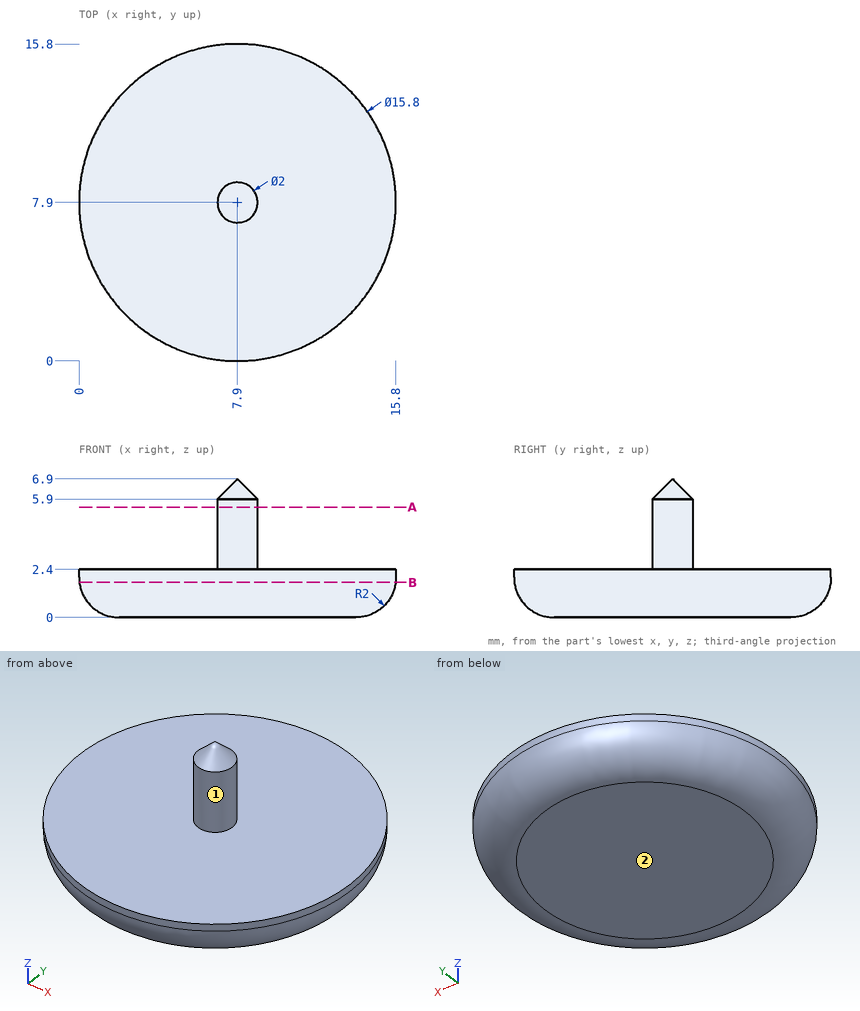
Design review of the part shown in the three views and the two pictorial views. Dimensions are in mm from the part's minimum x, y and z. A direction names the side the tool comes from. Round coordinates to 2 decimals unless told otherwise and drop trailing zeros. Loops run counter-clockwise (first coordinate to the right, second up) from the corner with the lowest first, then second, coordinate; pieces in that order, holes last. Notation, with made-up numbers: (37.5, -34.5) -> (71.5, -34.5) arc R30 cw to (71.5, -9.5) -> close; hole circle Ø10 at (26, 27.25). An arc over 180 degrees is marked (long way). Return JSON: item names as keys, results as strings.
(1) For pin 1 (3 mm diameter, centred on x = 13.5, y = 8.5, fed in from +Z); pin 2 (6 mm diameter, centred on x = 5, y = 2, fed in from -Z), all flat-tipped, find the tip position at first contact; note any pin that passes through.
Solved:
{"pin 1": "z = 2.4", "pin 2": "z = 0"}
(2) Add section B-B on z = 1.75. Write out the cut boundary in (x, y).
Solved:
{"outline": "circle Ø15.77 at (7.9, 7.9)"}
(3) For line 1 (Z direction, x = 9.25, y = 9.25); line 2 (X direction, y = 9.5, z = 1.5); line 3 (Y direction, x = 11.75, z = 1.25), list the stretches that pass through material, from the lowest coordinate up.
Solved:
{"line 1": "0 to 2.4", "line 2": "0.23 to 15.57", "line 3": "1.17 to 14.63"}
(4) For the marked faces 1 and 2, list the 3-axis set-ups (+Z, -Z, +X, -X, +Y, -Y) from which the entire face can be reached by the end or side of a thin tool; tool diameter is ignored.
Solved:
{"face 1": "+Z", "face 2": "-Z, +X, -X, +Y, -Y"}
(5) Add section A-A on z = 5.5. Write out the cut boundary in (x, y), plus the area to 3 significant figures.
Solved:
{"outline": "circle Ø2 at (7.9, 7.9)", "area": "3.14 mm2"}
